Source: CAD feature listing. Evaluate the final solid. Frame: model axes, mm. Face numbers are marked on the shaded views. A direction names the side the tool comes from. Give positions to 0.01 mm unless a question says otherwise; leave off trailing zeros. Loops run counter-clockwise (first coordinate to the right, second up) from the corner with the lowest first, then second, coordinate; pieces in that order, holes last.
Autodesk Inventor part; units mm, degrees
ref_plane "YZ Plane" through (0, 0, 0) normal (1, 0, 0) x (0, 1, 0)
ref_plane "XZ Plane" through (0, 0, 0) normal (0, 1, 0) x (-1, 0, 0)
ref_plane "XY Plane" through (0, 0, 0) normal (0, 0, 1) x (1, 0, 0)
sketch "Sketch1" plane through (0, 0, 0) normal (0, 1, 0) x (-1, 0, 0)
  circle A0 centre (0, 19.05) radius 2.2225
  circle A1 centre (-19.05, 0) radius 2.2225
  circle A2 centre (0, -19.05) radius 2.2225
  circle A3 centre (19.05, 0) radius 2.2225
  line L0 (0.635, 24.639) -> (0, 24.639)
  line L1 (0, 0) -> (0, 2.5439)
  line L2 (3.81, -19.812) -> (3.81, -16.51)
  line L3 (3.81, 16.51) -> (3.81, 19.812)
  line L4 (-19.812, 3.81) -> (-16.51, 3.81)
  line L5 (16.51, 3.81) -> (19.812, 3.81)
  line L6 (-3.81, 19.812) -> (-3.81, 16.51)
  line L7 (-3.81, -16.51) -> (-3.81, -19.812)
  line L8 (19.812, -3.81) -> (16.51, -3.81)
  line L9 (-16.51, -3.81) -> (-19.812, -3.81)
  arc A4 (3.81, 16.51) -> (16.51, 3.81) centre (16.51, 16.51) ccw
  arc A5 (16.51, -3.81) -> (3.81, -16.51) centre (16.51, -16.51) ccw
  arc A6 (-16.51, 3.81) -> (-3.81, 16.51) centre (-16.51, 16.51) ccw
  arc A7 (-3.81, -16.51) -> (-16.51, -3.81) centre (-16.51, -16.51) ccw
  line L10 (0, -3.81) -> (0, 0)
  line L11 (0, 3.81) -> (0, 0)
  line L12 (3.81, -19.812) -> (3.81, -16.51)
  line L13 (16.51, 3.81) -> (19.812, 3.81)
  line L14 (21.2725, 0) -> (16.8275, 0)
  line L15 (19.812, 3.81) -> (16.51, 3.81)
  line L16 (19.812, -3.81) -> (16.51, -3.81)
  line L17 (0, -3.81) -> (0.635, -3.81)
  line L18 (16.51, -3.81) -> (19.812, -3.81)
  line L19 (-19.812, -3.81) -> (-16.51, -3.81)
  line L20 (-3.81, -16.51) -> (-3.81, -19.812)
  line L21 (-3.81, -19.812) -> (-3.81, -16.51)
  line L22 (0, 0) -> (0.635, 0)
  line L23 (-0.635, 24.639) -> (0.635, 24.639)
  line L24 (0.635, 0) -> (0, 0)
  line L25 (-3.81, 16.51) -> (-3.81, 19.812)
  line L26 (22.987, -0.635) -> (22.987, 0.635)
  arc A8 (-24.0273, 24.8189) -> (-24.2117, 24.639) centre (0, 0) ccw
  line L27 (-19.812, 3.81) -> (-16.51, 3.81)
  line L28 (-3.81, 19.812) -> (-3.81, 16.51)
  line L29 (3.81, 19.812) -> (3.81, 16.51)
  line L30 (3.81, 19.812) -> (3.81, 16.51)
  line L31 (19.812, 3.81) -> (16.51, 3.81)
  line L32 (16.51, -3.81) -> (19.812, -3.81)
  line L33 (3.81, -16.51) -> (3.81, -19.812)
  line L34 (-19.812, -3.81) -> (-16.51, -3.81)
  line L35 (0, -3.81) -> (0.635, -3.81)
  line L36 (0.635, 3.81) -> (0, 3.81)
  line L37 (-16.51, 3.81) -> (-19.812, 3.81)
  arc A9 (19.812, -3.81) -> (22.987, -0.635) centre (19.812, -0.635) ccw
  arc A10 (22.987, 0.635) -> (19.812, 3.81) centre (19.812, 0.635) ccw
  line L38 (0, 0) -> (7.5297, 7.5297)
  line L39 (0, 0) -> (7.5297, -7.5297)
  circle A11 centre (0, 19.05) radius 2.2225
  line L40 (3.81, 16.51) -> (3.81, 19.812)
  line L41 (-3.81, 19.812) -> (-3.81, 16.51)
  line L42 (3.81, 16.51) -> (3.81, 19.812)
  line L43 (3.81, 19.812) -> (3.81, 16.51)
  line L44 (3.81, 19.812) -> (3.81, 16.51)
  line L45 (-3.81, 19.812) -> (-3.81, 16.51)
  line L46 (-3.81, 16.51) -> (-3.81, 19.812)
  line L47 (-3.81, 16.51) -> (-3.81, 19.812)
  line L48 (0, 21.2725) -> (0, 16.8275)
  arc A12 (-0.635, 22.987) -> (-3.81, 19.812) centre (-0.635, 19.812) ccw
  line L49 (-0.635, 22.987) -> (0.635, 22.987)
  arc A13 (3.81, 19.812) -> (0.635, 22.987) centre (0.635, 19.812) ccw
  arc A14 (3.81, 16.51) -> (16.51, 3.81) centre (16.51, 16.51) ccw
  arc A15 (-16.51, 3.81) -> (-3.81, 16.51) centre (-16.51, 16.51) ccw
  arc A16 (-16.51, 3.81) -> (-3.81, 16.51) centre (-16.51, 16.51) ccw
  line L50 (-3.81, 16.51) -> (-3.81, 19.812)
  arc A17 (-0.635, 22.987) -> (-3.81, 19.812) centre (-0.635, 19.812) ccw
  arc A18 (3.81, 19.812) -> (0.635, 22.987) centre (0.635, 19.812) ccw
  line L51 (0.635, 22.987) -> (-0.635, 22.987)
  arc A19 (3.81, 16.51) -> (16.51, 3.81) centre (16.51, 16.51) ccw
  line L52 (3.81, 19.812) -> (3.81, 16.51)
  arc A20 (-3.81, -16.51) -> (-16.51, -3.81) centre (-16.51, -16.51) ccw
  line L53 (-16.51, -3.81) -> (-19.812, -3.81)
  arc A21 (-22.987, -0.635) -> (-19.812, -3.81) centre (-19.812, -0.635) ccw
  arc A22 (-19.812, 3.81) -> (-22.987, 0.635) centre (-19.812, 0.635) ccw
  line L54 (-22.987, 0.635) -> (-22.987, -0.635)
  arc A23 (-16.51, 3.81) -> (-3.81, 16.51) centre (-16.51, 16.51) ccw
  line L55 (-19.812, 3.81) -> (-16.51, 3.81)
  arc A24 (16.51, -3.81) -> (3.81, -16.51) centre (16.51, -16.51) ccw
  line L56 (3.81, -16.51) -> (3.81, -19.812)
  arc A25 (0.635, -22.987) -> (3.81, -19.812) centre (0.635, -19.812) ccw
  arc A26 (-3.81, -19.812) -> (-0.635, -22.987) centre (-0.635, -19.812) ccw
  line L57 (-0.635, -22.987) -> (0.635, -22.987)
  arc A27 (-3.81, -16.51) -> (-16.51, -3.81) centre (-16.51, -16.51) ccw
  line L58 (-3.81, -19.812) -> (-3.81, -16.51)
  point P0 (19.05, 0)
  point P1 (0, -19.05)
  point P2 (-2.9852, -22.987)
  point P3 (-3.81, -29.2166)
  point P4 (0, 34.544)
  point P5 (-24.0273, 0)
  point P6 (0, -24.0273)
  point P7 (0, 19.05)
  point P8 (-7.5297, 7.5297)
  point P9 (7.5297, 7.5297)
  point P10 (-7.5297, -7.5297)
  point P11 (-7.5297, 7.5297)
  point P12 (7.5297, -7.5297)
  point P13 (-7.5297, -7.5297)
  dimension "d4" = 360
  dimension "d5" = 4.445
  dimension "d6" = 360
  dimension "d7" = 3.175
  dimension "d16" = 360
extrude "Extrusion1" add sketch "Sketch1" along normal blind 5.08
extrude "Extrusion2" add sketch "Sketch1" along normal blind 11.43 contours A0 L48 | L48 A0 | A1 | A2 | A3 L14 picked at (18.3725, -0.5216)
extrude "Extrusion3" add sketch "Sketch1" along normal blind 11.43 contours L14 A3 picked at (19.7275, 0.5216)
sketch "Sketch2" plane through (0, 5.08, 0) normal (0, 1, 0) x (1, 0, 0)
  circle A0 centre (0, 0) radius 2.8575
  dimension "d18" = 5.715
extrude "Extrusion4" cut sketch "Sketch2" against normal blind 11.43
sketch "Sketch3" plane through (0, 0, 0) normal (0, -1, 0) x (1, 0, 0)
  circle A0 centre (0, 0) radius 2.8575
  circle A1 centre (0, 0) radius 5.3975
  dimension "d21" = 2.54
  dimension "d22" = 5.715
extrude "Extrusion5" add sketch "Sketch3" along normal blind 5.08
sketch "Sketch4" plane through (0, 5.08, 0) normal (0, 1, 0) x (1, 0, 0)
  circle A0 centre (0, 0) radius 3.81
  dimension "d25" = 7.62
extrude "Extrusion6" cut sketch "Sketch4" against normal blind 3.81
sketch "Sketch5" plane through (0, 1.27, 0) normal (0, 1, 0) x (1, 0, 0)
  circle A0 centre (0, 0) radius 3.175
  dimension "d28" = 6.35
extrude "Extrusion7" cut sketch "Sketch5" against normal blind 50.8
sketch "Sketch6" plane through (0, 1.27, 0) normal (0, 1, 0) x (1, 0, 0)
  circle A0 centre (0, 0) radius 1.905
  circle A1 centre (0, 0) radius 3.175
  dimension "d31" = 3.81
extrude "Extrusion8" add sketch "Sketch6" against normal blind 2.54
sketch "Sketch7" plane through (0, -5.08, 0) normal (0, -1, 0) x (1, 0, 0)
  circle A0 centre (0, 0) radius 3.175
  circle A1 centre (0, 0) radius 5.3975
extrude "Extrusion9" add sketch "Sketch7" along normal blind 2.54
properties part number "planetaryGearMt2"
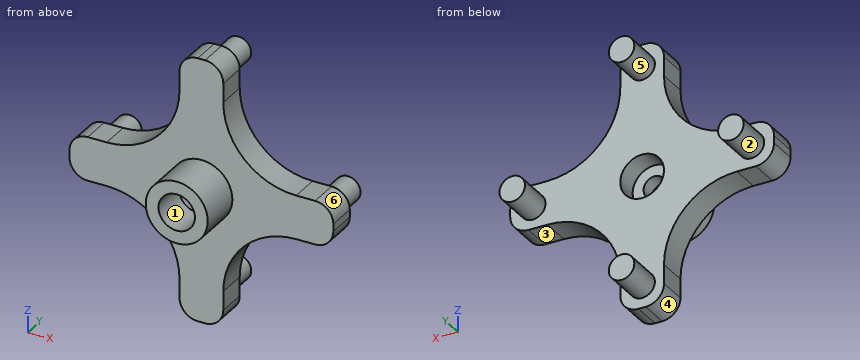
(1) Section B-B, the plane x = 0. Return the cut outline in (y, z) (1 decimal).
A:
outline: (-7.6, -5.4) - (0, -5.4) - (0, -23) - (5.1, -23) - (5.1, -21.3) - (11.4, -21.3) - (11.4, -16.8) - (5.1, -16.8) - (5.1, -3.8) - (1.3, -3.8) - (1.3, -1.9) - (-1.3, -1.9) - (-1.3, -3.2) - (-7.6, -3.2) - close; (-7.6, 3.2) - (-1.3, 3.2) - (-1.3, 1.9) - (1.3, 1.9) - (1.3, 3.8) - (5.1, 3.8) - (5.1, 16.8) - (11.4, 16.8) - (11.4, 21.3) - (5.1, 21.3) - (5.1, 23) - (0, 23) - (0, 5.4) - (-7.6, 5.4) - close
(2) First-contact query: pin 1 (1.7 mm diameter, centred on x = 18.5, y = 1.5, fed in from +Z); pin 2 (1.7 mm diameter, centred on y = 1.5, z = -18.5, fed in from -X); pin 3 (1.7 mm diameter, centred on y = 2.5, z = 18.5, fed in from +X); pin 4 (2 mm diameter, centred on x = -15, y = 7.5, fed in from +Z). Flat tips, straight axial feed; report the tip coordinate or a pass-through.
A:
pin 1: stops at z = 3.81
pin 2: stops at x = -3.81
pin 3: stops at x = 3.81
pin 4: passes through
(3) Section D-D, the plane x = -19.05. Return the cut outline in (y, z), then the cut area to 3 significant figures.
A:
outline: (0, -3.81) - (5.08, -3.81) - (5.08, -2.22) - (11.43, -2.22) - (11.43, 2.22) - (5.08, 2.22) - (5.08, 3.81) - (0, 3.81) - close
area: 66.9 mm2
(4) Mould query, pull axis Z, two halves, no side actions, for the marked faces 4, 5 and 6. Classes: pulls with the +Z half, pulls with the -Z half, needs draft (parallel to the pull), parting line crosses it, or undercut.
A:
face 4: pulls with the -Z half
face 5: undercut
face 6: pulls with the +Z half
(5) Section C-C, the plane y = 4.5. Return the cut outline in (x, z) (3 decimals).
A:
outline: (-22.987, -0.635) arc R3.175 ccw to (-19.812, -3.81) - (-16.51, -3.81) arc R12.7 cw to (-3.81, -16.51) - (-3.81, -19.812) arc R3.175 ccw to (-0.635, -22.987) - (0.635, -22.987) arc R3.175 ccw to (3.81, -19.812) - (3.81, -16.51) arc R12.7 cw to (16.51, -3.81) - (19.812, -3.81) arc R3.175 ccw to (22.987, -0.635) - (22.987, 0.635) arc R3.175 ccw to (19.812, 3.81) - (16.51, 3.81) arc R12.7 cw to (3.81, 16.51) - (3.81, 19.812) arc R3.175 ccw to (0.635, 22.987) - (-0.635, 22.987) arc R3.175 ccw to (-3.81, 19.812) - (-3.81, 16.51) arc R12.7 cw to (-16.51, 3.81) - (-19.812, 3.81) arc R3.175 ccw to (-22.987, 0.635) - close; hole circle Ø7.62 at (0, 0)
(6) Ray query, line 1 along Z through (x, y) = (0, 3.9); line 2 along Z through (x, y) = (0, -0.6) (1 decimal). Return the intervals inside material, ascending.
A:
line 1: z = -22.99 to -3.81, 3.81 to 22.99
line 2: z = -5.4 to -1.9, 1.9 to 5.4
(7) Reachability of the marked faces 1, 2 and 3 from +Z, -Z, +X, -X, +Y, -Y: full face, straight path, thin tool, end or side. Return the list, or none.
A:
face 1: -Y
face 2: +Y
face 3: -Z, +X, +Y, -Y
(8) Section A-A, the plane z = 0. Return the cut outline in (x, y) (1 decimal).
A:
outline: (-23, 0) - (-5.4, 0) - (-5.4, -7.6) - (-3.2, -7.6) - (-3.2, -1.3) - (-1.9, -1.3) - (-1.9, 1.3) - (-3.8, 1.3) - (-3.8, 5.1) - (-16.8, 5.1) - (-16.8, 11.4) - (-21.3, 11.4) - (-21.3, 5.1) - (-23, 5.1) - close; (1.9, -1.3) - (3.2, -1.3) - (3.2, -7.6) - (5.4, -7.6) - (5.4, 0) - (23, 0) - (23, 5.1) - (21.3, 5.1) - (21.3, 11.4) - (16.8, 11.4) - (16.8, 5.1) - (3.8, 5.1) - (3.8, 1.3) - (1.9, 1.3) - close
